Verification items for the finished model (mm, model axes). Round coordinates to 2 decimals unless told otherwise and drop trailing zeros. Loops run counter-clockwise (first coordinate to the right, second up) from the corner with the lowest first, then second, coordinate; pieces in that order, holes last. Notation, with made-up numbers: M 38,71 L 51,71 A34 ccw 51,110 Z; hole C 75.5,-22.5 d9. An arc over 180 degrees is marked long. Answer as CSV lines item,"result".
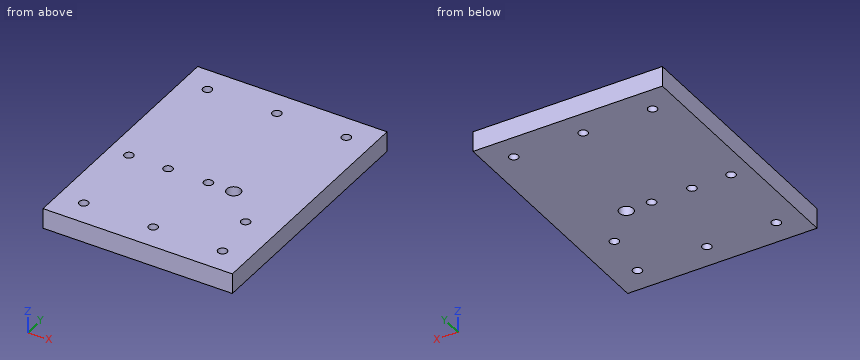
```python
from build123d import *

# Parameters (mm, degrees)
BOX_W         = 75
BOX_H         = 100
BOX_DEPTH     = 8
SKETCH_R      = 1.8
HOLE_DEPTH    = 8.001
SKETCH001_R   = 1.8
HOLE001_DEPTH = 25
SKETCH003_R   = 2.75
HOLE002_DEPTH = 8.001


with BuildPart() as part:
    # Box → Box (join)
    with BuildSketch(Plane.XY):
        with Locations((37.5, 50)):
            Rectangle(BOX_W, BOX_H)
    extrude(amount=BOX_DEPTH)

    # Sketch (on Face5 of Box) → Hole (cut, through all)
    with BuildSketch(Plane(origin=(0, 0, 0), x_dir=(1, 0, 0), z_dir=(0, 0, -1))):
        with Locations((10, -10)):
            Circle(SKETCH_R)
        with Locations((37.5, -10)):
            Circle(SKETCH_R)
        with Locations((65, -10)):
            Circle(SKETCH_R)
        with Locations((10, -90)):
            Circle(SKETCH_R)
        with Locations((37.5, -90)):
            Circle(SKETCH_R)
        with Locations((65, -90)):
            Circle(SKETCH_R)
    extrude(amount=-HOLE_DEPTH, mode=Mode.SUBTRACT)

    # Sketch001 (on Face5 of Hole) → Hole001 (cut)
    with BuildSketch(Plane(origin=(0, 0, 0), x_dir=(1, 0, 0), z_dir=(0, 0, -1))):
        with Locations((39.5, -42.5)):
            Circle(SKETCH001_R)
        with Locations((23.5, -42.5)):
            Circle(SKETCH001_R)
        with Locations((8, -42.5)):
            Circle(SKETCH001_R)
        with Locations((62.5, -29)):
            Circle(SKETCH001_R)
    extrude(amount=-HOLE001_DEPTH, mode=Mode.SUBTRACT)

    # Sketch003 (on Face5 of Hole001) → Hole002 (cut, through all)
    with BuildSketch(Plane(origin=(0, 0, 0), x_dir=(1, 0, 0), z_dir=(0, 0, -1))):
        with Locations((49.5, -42.5)):
            Circle(SKETCH003_R)
    extrude(amount=-HOLE002_DEPTH, mode=Mode.SUBTRACT)


solid = part.part
```
1) Section check C-C (x = 23.5). Record the cut outline in (y, z).
Here are the results:
outline,"M 0,0 L 40.7,0 L 40.7,8 L 0,8 Z; M 44.3,0 L 100,0 L 100,8 L 44.3,8 Z"
2) Material ranges on probe 1 along Y at (x, z) = (65, 4.75); probe 2 along X at (y, z) = (42.5, 2); probe 3 along X at (y, z) = (90, 2.75), recorded low to high.
Here are the results:
probe 1,"y = 0 to 8.2, 11.8 to 88.2, 91.8 to 100"
probe 2,"x = 0 to 6.2, 9.8 to 21.7, 25.3 to 37.7, 41.3 to 46.75, 52.25 to 75"
probe 3,"x = 0 to 8.2, 11.8 to 35.7, 39.3 to 63.2, 66.8 to 75"
3) Section check A-A (y = 29). Record the cut outline in (x, z).
Here are the results:
outline,"M 0,0 L 60.7,0 L 60.7,8 L 0,8 Z; M 64.3,0 L 75,0 L 75,8 L 64.3,8 Z"
4) Section check D-D (z = 3). State how many separate pieces and enclosed holes the cut face has, plus the area to 3 significant figures.
Here are the results:
separate pieces,"1"
enclosed holes,"11"
area,"7,370 mm^2"
5) Section check B-B (y = 90). Record the cut outline in (x, z).
Here are the results:
outline,"M 0,0 L 8.2,0 L 8.2,8 L 0,8 Z; M 11.8,0 L 35.7,0 L 35.7,8 L 11.8,8 Z; M 39.3,0 L 63.2,0 L 63.2,8 L 39.3,8 Z; M 66.8,0 L 75,0 L 75,8 L 66.8,8 Z"
6) Go/stop test with a flat-tipped pin: pin 1 (3 mm diameter, centred on x = 23.5, y = 42.5, fed in from +Z). Record where the tip stops, or that it passes through.
Here are the results:
pin 1,"passes through"
